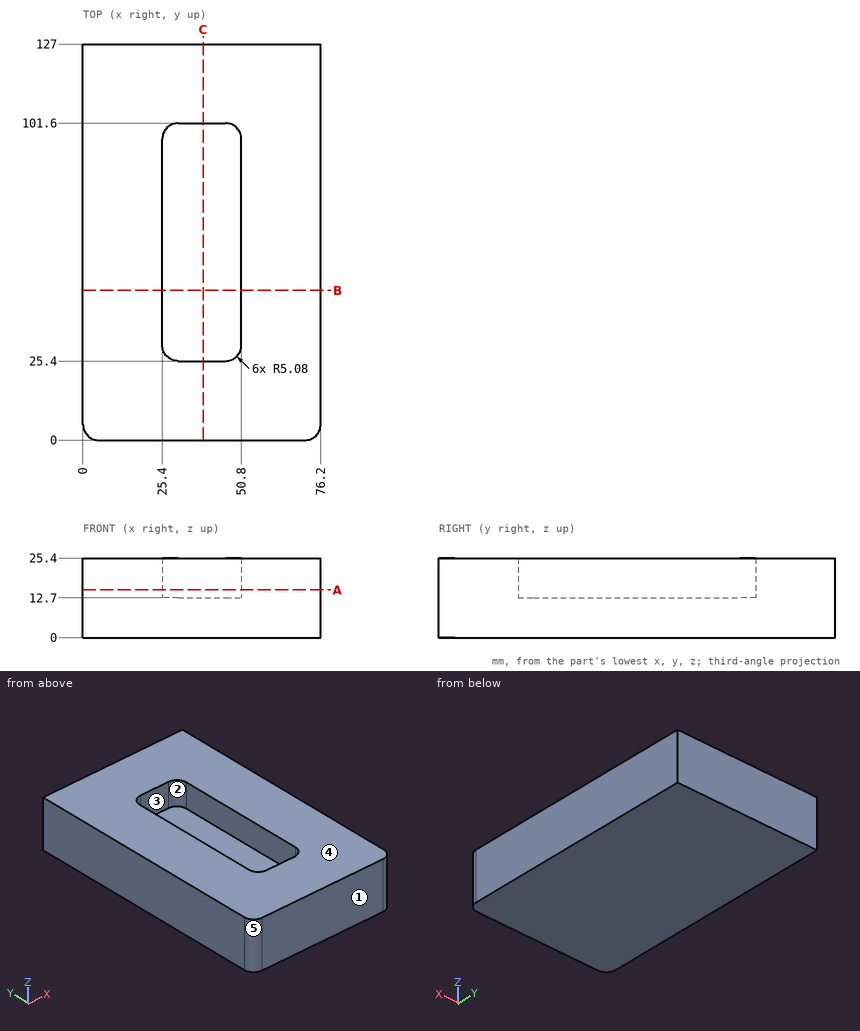
Design review of the part shown in the three views and the two pictorial views. Dimensions are in mm from the part's minimum x, y and z. A direction names the side the tool comes from. Coordinates: 2 decimals unless noted, no trailing zeros. Order: outer loops, then holes, each group sorted by start corner. A loop starts at its lowest first (then second) coordinate and runs counter-clockwise, first axis right, second up.
1) Take a section at A-A, the plane z = 15.25. Give the boundary of the cut face in (x, y), and give its area (3 significant figures).
2) Take a section at B-B, the plane y = 48. Give the boundary of the cut face in (x, z), and give its area (3 significant figures).
3) For the marked faces 1 and 2, list the 3-axis set-ups (+Z, -Z, +X, -X, +Y, -Y) from which the entire face can be reached by the end or side of a thin tool; tool diameter is ignored.
4) Wall thickness on line 1 along Y through (x, z) = (33.5, 15.5); line 2 along X through (y, z) = (35, 21); line 3 along Y through (x, z) = (72, 9.25): over which ranges is each line inside the solid? List them lowest first.
5) Clearance check with a flat-ended pin moving along its axis: pin 1 (12.5 mm diameter, centred on x = 36, y = 51.5, fed in from +Z). State where the tip first meets the part, or that it passes through.
6) Mouldability with a two-part tool opening along Y and no side actions: class the marked faces 3, 4 and 5 as +Y half, -Y half, draft (parallel to the pull), parting line (faces both ways), or undercut.
7) Take a section at C-C, the plane x = 38.5. Give the boundary of the cut face in (y, z).
Returned:
1. outline: (0, 5.08) arc R5.08 ccw to (5.08, 0) - (71.12, 0) arc R5.08 ccw to (76.2, 5.08) - (76.2, 127) - (0, 127) - close; hole (25.4, 30.48) arc R5.08 ccw to (30.48, 25.4) - (45.72, 25.4) arc R5.08 ccw to (50.8, 30.48) - (50.8, 96.52) arc R5.08 ccw to (45.72, 101.6) - (30.48, 101.6) arc R5.08 ccw to (25.4, 96.52) - close
1. area: 7,750 mm2
2. outline: (0, 0) - (76.2, 0) - (76.2, 25.4) - (50.8, 25.4) - (50.8, 12.7) - (25.4, 12.7) - (25.4, 25.4) - (0, 25.4) - close
2. area: 1,610 mm2
3. face 1: +Z, -Z, +X, -X, -Y
3. face 2: +Z
4. line 1: y = 0 to 25.4, 101.6 to 127
4. line 2: x = 0 to 25.4, 50.8 to 76.2
4. line 3: y = 0.08 to 127
5. pin 1: stops at z = 12.7
6. face 3: undercut
6. face 4: draft
6. face 5: -Y half
7. outline: (0, 0) - (127, 0) - (127, 25.4) - (101.6, 25.4) - (101.6, 12.7) - (25.4, 12.7) - (25.4, 25.4) - (0, 25.4) - close
